from build123d import *

# Parameters (mm, degrees)
F0_W     = 25.4
F0_H     = 63.5
F1_DEPTH = 25.4
F3_DEPTH = 25.4
F4_R     = 4.7625
F5_DEPTH = 1.27
F7_DEPTH = 1.27


with BuildPart() as f1:
    # F0 (on Top) → F1 (new body)
    with BuildSketch(Plane.XY):
        Polygon((95.231725046, 52.6741128501), (-82.568274954, 52.6741128501), (-82.568274954, 14.5741128501), (-57.168274954, 14.5741128501), (69.831725046, 14.5741128501), (95.231725046, 14.5741128501), align=None)
        with Locations((-69.868274954, -17.1758871499)):
            Rectangle(F0_W, F0_H)
        with Locations((82.531725046, -17.1758871499)):
            Rectangle(F0_W, F0_H)
    extrude(amount=F1_DEPTH)

    # F2 (on face) → F3 (cut)
    with BuildSketch(Plane.XY.offset(25.4)):
        Polygon((-104.4803282541, 40.2830914566), (-99.053036825, 22.9674405237), (-44.5216608105, 67.1611169851), (-66.7477198675, 76.2066116208), align=None)
        Polygon((81.9489609954, 70.5137167564), (63.5293972251, 62.1673528543), (115.3344315049, 19.8599052123), (133.17838577, 37.4160547248), align=None)
    extrude(amount=-F3_DEPTH, mode=Mode.SUBTRACT)

    # F4 (on face) → F5 (join)
    with BuildSketch(Plane.XY.offset(25.4)):
        with Locations((-70.5124139786, -17.1758871499)):
            Circle(F4_R)
        with Locations((81.896725046, -17.1758871499)):
            Circle(F4_R)
    extrude(amount=F5_DEPTH)

    # F6 (on face) → F7 (join)
    with BuildSketch(Plane(origin=(0, 0, 0), x_dir=(1, 0, 0), z_dir=(0, 0, -1))):
        with BuildLine():
            ThreePointArc((82.531725046, 21.9383871499), (77.769225046, 17.1758871499), (82.531725046, 12.4133871499))
            Line((82.531725046, 12.4133871499), (82.531725046, 21.9383871499))
        make_face()
        with BuildLine():
            Line((82.531725046, 21.9383871499), (82.531725046, 12.4133871499))
            ThreePointArc((82.531725046, 12.4133871499), (85.8993210914, 13.8082911045), (87.294225046, 17.1758871499))
            ThreePointArc((87.294225046, 17.1758871499), (85.8993210914, 20.5434831953), (82.531725046, 21.9383871499))
        make_face()
        with BuildLine():
            ThreePointArc((-70.0870901346, 12.4133871499), (-66.7194940892, 13.8082911045), (-65.3245901346, 17.1758871499))
            ThreePointArc((-65.3245901346, 17.1758871499), (-66.7194940892, 20.5434831953), (-70.0870901346, 21.9383871499))
            Line((-70.0870901346, 21.9383871499), (-70.0870901346, 12.4133871499))
        make_face()
        with BuildLine():
            Line((-70.0870901346, 12.4133871499), (-70.0870901346, 21.9383871499))
            ThreePointArc((-70.0870901346, 21.9383871499), (-74.8495901346, 17.1758871499), (-70.0870901346, 12.4133871499))
        make_face()
    extrude(amount=F7_DEPTH)


solid = f1.part
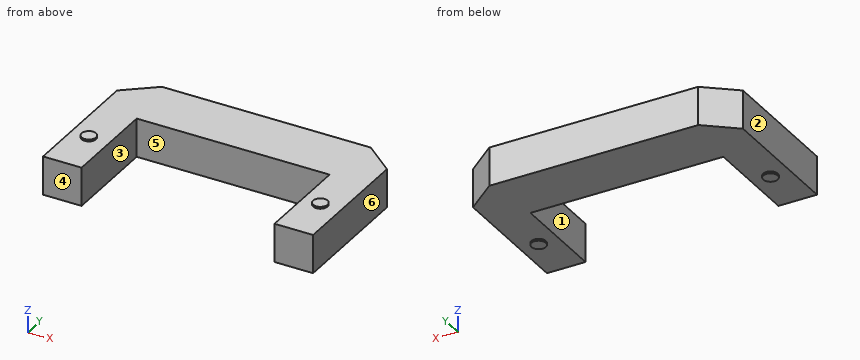
Design review of the part built by this model. Coordinates are the model's own, in mm. Face numbers are marked on the shaded views. A direction names the side the tool comes from. Round coordinates to 2 decimals unless told otherwise and drop trailing zeros. Write each loop counter-clockwise with the first axis right and the second up, starting at its lowest first coordinate (ties: lowest second). Pieces come first, ordered by that corner, then holes.
Item 1: Consider section D-D on y = 40.5. Give the boundary of the cut face in (x, z), and give its area (3 significant figures).
Item 2: Consider section B-B on z = 3. Give the boundary of the cut face in (x, y).
Item 3: Consider section A-A on y = -9.5. Give the boundary of the cut face in (x, z), and give its area (3 significant figures).
Item 4: Consider section C-C on x = -68. Give the boundary of the cut face in (y, z).
Item 5: Wall thickness on L1, parallel to X at y = -30.5, z = 4.75; L2, parallel to Z at x = -43.5, y = 43; L3, parallel to Y at x = 1, z = 1: over which ranges is each line inside the solid? List them lowest first.
Item 6: For the marked faces 5 and 6, list the 3-axis set-ups (+Z, -Z, +X, -X, +Y, -Y) from which the entire face can be reached by the end or side of a thin tool; tool diameter is ignored.
Item 7: Draft analysis for pull direction X (two halves, no side actions). For the marked faces 1, 2, 3 and 4, state which applies: released by +X, released by -X, zero draft, split by the parting line, or undercut.
Item 8: For pin 1 Ø1.5 at (x, z) = (-27.5, 3) entering from -Y; pin 2 Ø5 at (x, y) = (43, 41.5) entering from +Z; pin 3 Ø12 at (x, y) = (-34.5, 41) entering from -Z, all flat-tipped, find the tip position at first contact; note any pin that passes through.
Check values:
1. outline: (-77.42, 0) - (90.06, 0) - (90.06, 25.4) - (-77.42, 25.4) - close
1. area: 4,250 mm2
2. outline: (-82.57, -48.93) - (-57.17, -48.93) - (-57.17, 14.57) - (69.83, 14.57) - (69.83, -48.93) - (95.23, -48.93) - (95.23, 36.28) - (75.15, 52.67) - (-62.4, 52.67) - (-82.57, 36.33) - close
3. outline: (-82.57, 0) - (-57.17, 0) - (-57.17, 25.4) - (-82.57, 25.4) - close; (69.83, 0) - (95.23, 0) - (95.23, 25.4) - (69.83, 25.4) - close
3. area: 1,290 mm2
4. outline: (-48.93, 0) - (-21.46, 0) - (-21.46, -1.27) - (-12.9, -1.27) - (-12.9, 0) - (48.13, 0) - (48.13, 25.4) - (-13.13, 25.4) - (-13.13, 26.67) - (-21.22, 26.67) - (-21.22, 25.4) - (-48.93, 25.4) - close
5. L1: x = -82.57 to -57.17, 69.83 to 95.23
5. L2: z = 0 to 25.4
5. L3: y = 14.57 to 52.67
6. face 5: +Z, -Z, -Y
6. face 6: +Z, -Z, +X, +Y, -Y
7. face 1: undercut
7. face 2: released by -X
7. face 3: undercut
7. face 4: zero draft
8. pin 1: stops at y = 14.57
8. pin 2: stops at z = 25.4
8. pin 3: stops at z = 0
